Geometry: final body of the model. Coordinates: model frame, mm. Round coordinates to 2 decimals unless told otherwise and drop trailing zeros. Write each loop counter-clockwise with the first axis right and the second up, starting at its lowest first coordinate (ties: lowest second). Pieces come first, ordered by that corner, then holes. Notation, with made-up numbers: (-7.75, 63.25) -> (48.25, 63.25) arc R20 ccw to (48.25, 100.25) -> close; hole circle Ø7 at (39, -25.5). An arc over 180 degrees is marked (long way). Use one line per item in the form item = value. Start each with the question number.
1. Draft query along X for faces 1 (the face through (7, 3, -2.5)), 2 (the face through (-10.135, 3.042, -0.141)), 3 (the face through (11.748, 3.042, 1.787)). Return one class per face: pulls with the +X half, pulls with the -X half, needs draft (parallel to the pull), parting line crosses it, or undercut.
2. Cut plane D-D, the plane x = 3. Return the cut outline in (y, z), plus the area to 3 significant figures.
3. Cut plane A-A, the plane x = 9.5. Return the cut outline in (y, z), plus the area to 3 significant figures.
4. Pin query (flat end, axial travel): pin 1 Ø3 at (x, z) = (9.5, 0) entering from +Y. Return the tip coordinate at first contact, or that it passes through.
5. Cut plane B-B, the plane y = 1.5. State how many separate pieces and enclosed holes the cut face has, plus the area to 3 significant figures.
6. Cut plane C-C, the plane x = -6.75. Return the cut outline in (y, z).
7. Line query: L1, parallel to X at y = 4.05, z = 0; L2, parallel to X at y = 5.25, z = -0.55; L3, parallel to X at y = 1, z = -1.1. Output: solid intervals per line, ascending.
```python
from build123d import *

# Parameters (mm, degrees)
SKETCH_1_W          = 25
SKETCH_1_H          = 5
EXTRUDE_1_DEPTH     = 6
SKETCH_2_R          = 1.6
SKETCH_2_R_2        = 0.65
CUT_EXTRUDE_1_DEPTH = 10
FILLET_1_R          = 2.5
CUT_EXTRUDE_2_DEPTH = 7


with BuildPart() as part:
    # 草图1 → 凸台-拉伸1 (new body)
    with BuildSketch(Plane(origin=(0, 0, 0), x_dir=(1, 0, 0), z_dir=(0, 1, 0))):
        Rectangle(SKETCH_1_W, SKETCH_1_H)
    extrude(amount=EXTRUDE_1_DEPTH)

    # 草图2 → 切除-拉伸1 (cut)
    with BuildSketch(Plane(origin=(0, 6, 0), x_dir=(1, 0, 0), z_dir=(0, 1, 0))):
        with Locations(Location((9.5, 0, 0), (0, 0, 270))):
            Circle(SKETCH_2_R)
        with Locations(Location((-9.5, 0, 0), (0, 0, 270))):
            Circle(SKETCH_2_R_2)
    extrude(amount=-CUT_EXTRUDE_1_DEPTH, mode=Mode.SUBTRACT)

    # 圆角1
    fillet_1_edges = [part.edges().sort_by_distance(p)[0] for p in [
        (12.5, 3, 2.5),
        (12.5, 3, -2.5),
        (-12.5, 3, 2.5),
        (-12.5, 3, -2.5),
    ]]
    fillet(fillet_1_edges, radius=FILLET_1_R - 0.0001)  # a hair under: the kernel refuses the full size

    # 草图3 → 切除-拉伸2 (cut)
    with BuildSketch(Plane(origin=(0, 6, 0), x_dir=(1, 0, 0), z_dir=(0, 1, 0))):
        with BuildLine():
            Line((-9.571202172, 1.998732161), (4.5, 2.5))
            Line((4.5, 2.5), (-10, 2.5))
            ThreePointArc((-10, 2.5), (-11.767766953, 1.767766953), (-12.5, 0))
            ThreePointArc((-12.5, 0), (-11.767766953, -1.767766953), (-10, -2.5))
            Line((-10, -2.5), (4.5, -2.5))
            Line((4.5, -2.5), (-9.571202172, -1.998732161))
            ThreePointArc((-9.571202172, -1.998732161), (-11.5, 0), (-9.571202172, 1.998732161))
        make_face()
    extrude(amount=-CUT_EXTRUDE_2_DEPTH, mode=Mode.SUBTRACT)


with BuildPart() as cut_extrude_2_kept_piece:
    # of the separate pieces the step leaves, the one the design keeps (cut_extrude_2_pieces_kept)
    add(part.part.solids().sort_by_distance((4.5, 0, -2.5))[0])


solid = cut_extrude_2_kept_piece.part
```
Outcome:
q1.face_1 = needs draft
q1.face_2 = undercut
q1.face_3 = pulls with the +X half
q2.outline = (0, -2.45) -> (6, -2.45) -> (6, 2.45) -> (0, 2.45) -> close
q2.area = 29.4 mm^2
q3.outline = (0, -2.5) -> (6, -2.5) -> (6, -1.6) -> (0, -1.6) -> close; (0, 1.6) -> (6, 1.6) -> (6, 2.5) -> (0, 2.5) -> close
q3.area = 10.8 mm^2
q4.pin_1 = through
q5.separate_pieces = 1
q5.enclosed_holes = 2
q5.area = 97.2 mm^2
q6.outline = (0, -2.1) -> (6, -2.1) -> (6, 2.1) -> (0, 2.1) -> close
q7.L1 = -11.5 to -10.15, -8.85 to 7.9, 11.1 to 12.5
q7.L2 = -11.42 to -9.85, -9.15 to 8, 11 to 12.44
q7.L3 = -11.17 to 8.34, 10.66 to 12.25
